Here's how the part is built. I have some questions about the finished solid (model axes, mm). Face numbers are marked on the shaded views. A direction names the side the tool comes from. Coordinates: 2 decimals unless noted, no trailing zeros. Loops run counter-clockwise (first coordinate to the right, second up) from the corner with the lowest first, then second, coordinate; pieces in that order, holes last. Notation, with made-up numbers: M 64.25,-1 L 109.25,-1 A20 cw 109.25,4 Z; hole C -39,54 d9. An arc over 180 degrees is marked long. Use CSV: the item, a comma, the result in double quotes. Start each with the question number.
Q1. If we section it at A-A (x = -6.35): Please give me the cut outline in (y, z) (3 decimals), and give its area (3 significant figures).
Q2. If we section it at C-C (x = -2): Please give me the cut outline in (y, z) (3 decimals).
Q3. If we mould it in two halves opening along Z, with no side actions, what happens to the marked faces 1, 2 and 3? For each: +Z half, -Z half, draft (parallel to the pull), parting line (faces both ways), or undercut.
Q4. If we section it at D-D (x = 8.5): Please give me the cut outline in (y, z) (3 decimals).
Q5. For pin 1 Ø5 at (x, y) = (12.7, 11.11) entering from -Z (3 decimals); pin 2 Ø3 at (x, z) = (10.5, 1.5) entering from -Y; pin 3 Ø4 at (x, z) = (-8, 2) entering from -Y, each with a flat end and sliding along its axis, tell me the tip position at first contact or that it passes through.
Q6. Which directions (+Z, -Z, +X, -X, +Y, -Y) give clear straight access to the entire face, cutting with the end or side of a thin tool? Please do the marked faces 4, 5 and 6.
Q7. Please list where these lines run through material, in increasing order: probe 1 along Z at (x, y) = (16.5, -4.5) (3 decimals); probe 2 along Y at (x, z) = (-9, 5.75); probe 3 along Y at (x, z) = (-10.5, -0.5) (3 decimals). Write a range as [from, to].
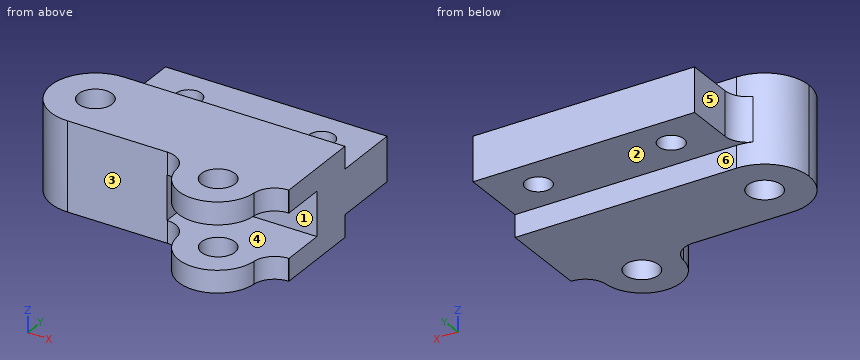
from build123d import *

# Parameters (mm, degrees)
SKETCH1_W                             = 38.1
SKETCH1_H                             = 12.699999999999998
BOSS_EXTRUDE1_DEPTH                   = 6.35
BOSS_EXTRUDE2_DEPTH                   = 3.175
F_6_CLEARANCE_HOLE1_D                 = 3.6576
F_3_16_0_1875_CLEARANCE_DOWEL_HOLE1_D = 4.826
CUT_EXTRUDE3_DEPTH                    = 3.1496
CUT_EXTRUDE3_DEPTH_BACK               = 3.175
SKETCH8_W                             = 17.4625
SKETCH8_H                             = 14.287499999999998
FILLET2_RADIUS                        = 5.55625
FILLET2_LENGTH                        = 3.2004
FILLET3_RADIUS                        = 5.55625
FILLET3_LENGTH                        = 3.175
FILLET5_R                             = 3.175
FILLET7_R                             = 6.35
FILLET8_R                             = 3.175


# Some blends are built 0.0001 mm under size
with BuildPart() as part:
    # Sketch1 → Boss-Extrude1 (new, symmetric)
    with BuildSketch(Plane.XY):
        Polygon((15.875, -14.287499999999998), (15.875, -6.349999999999994), (4.762500000000001, -6.35), (4.762500000000001, -14.287499999999996), align=None)
        Rectangle(SKETCH1_W, SKETCH1_H)
    extrude(amount=BOSS_EXTRUDE1_DEPTH, both=True)

    # Sketch2 → Boss-Extrude2 (add, symmetric)
    with BuildSketch(Plane.XY):
        Polygon((19.05, 6.35), (-12.7, 6.349999999999996), (-12.7, 15.874999999999996), (19.05, 15.875), align=None)
    extrude(amount=BOSS_EXTRUDE2_DEPTH, both=True)

    # #6 Clearance Hole1 (through all)
    with Locations(Plane.XY.offset(3.175)):
        with Locations((-6.35, 11.1125), (12.7, 11.1125)):
            Hole(F_6_CLEARANCE_HOLE1_D / 2)

    # 3/16 (0.1875) Clearance Dowel Hole1 (through all)
    with Locations(Plane.XY.offset(6.35)):
        with Locations((-12.7, 0), (10.31875, -8.5725)):
            Hole(F_3_16_0_1875_CLEARANCE_DOWEL_HOLE1_D / 2)

    # Sketch8 → Cut-Extrude3 (cut, two sides: drawn at the far end of the back side and taken through both)
    with BuildSketch(Plane.XY.offset(-CUT_EXTRUDE3_DEPTH_BACK)):
        with Locations((10.318750000000001, -7.143749999999999)):
            Rectangle(SKETCH8_W, SKETCH8_H)
    extrude(amount=CUT_EXTRUDE3_DEPTH + CUT_EXTRUDE3_DEPTH_BACK, mode=Mode.SUBTRACT)

    # Fillet2: full round fillet: the end face becomes a half cylinder, R = half its width
    fillet2_face = Plane((10.31875, -14.2875, 4.7498), x_dir=(0, 0, 1), z_dir=(0, -1, 0))  # on the end face: x along it, z out of the body
    fillet2_slab = fillet2_face.offset(-FILLET2_RADIUS / 2) * Box(FILLET2_LENGTH, 2 * FILLET2_RADIUS, FILLET2_RADIUS, mode=Mode.PRIVATE)  # the body's end, R deep
    fillet2_round = Plane((10.31875, -8.73125, 4.7498), x_dir=(0, -1, 0), z_dir=(0, 0, 1)) * Cylinder(FILLET2_RADIUS, FILLET2_LENGTH, mode=Mode.PRIVATE)  # its axis R under the face
    add(fillet2_slab - fillet2_round, mode=Mode.SUBTRACT)

    # Fillet3: full round fillet: the end face becomes a half cylinder, R = half its width
    fillet3_face = Plane((10.31875, -14.2875, -4.7625), x_dir=(0, 0, 1), z_dir=(0, -1, 0))  # on the end face: x along it, z out of the body
    fillet3_slab = fillet3_face.offset(-FILLET3_RADIUS / 2) * Box(FILLET3_LENGTH, 2 * FILLET3_RADIUS, FILLET3_RADIUS, mode=Mode.PRIVATE)  # the body's end, R deep
    fillet3_round = Plane((10.31875, -8.73125, -4.7625), x_dir=(0, -1, 0), z_dir=(0, 0, 1)) * Cylinder(FILLET3_RADIUS, FILLET3_LENGTH, mode=Mode.PRIVATE)  # its axis R under the face
    add(fillet3_slab - fillet3_round, mode=Mode.SUBTRACT)

    # Fillet5
    fillet5_edges = [part.edges().sort_by_distance(p)[0] for p in [
        (15.875, -6.349999999999997, 4.7498),
        (15.875, -6.349999999999997, -4.762499999999999),
        (4.762500000000001, -6.349999999999998, -4.762499999999999),
        (4.762500000000001, -6.349999999999998, 4.7498),
    ]]
    fillet(fillet5_edges, radius=FILLET5_R - 0.0001)  # a hair under: the kernel refuses the full size

    # Fillet7
    fillet7_edges = [part.edges().sort_by_distance(p)[0] for p in [
        (-19.05, -6.35, 0),
        (-19.05, 6.35, 0),
    ]]
    fillet(fillet7_edges, radius=FILLET7_R - 0.0001)  # a hair under: the kernel refuses the full size

    # Fillet8
    # the kernel refuses this fillet: 3.175 mm, written as the material it adds along each edge
    with BuildSketch(Plane(origin=(-12.7, 6.349999999999996, 3.175), x_dir=(-0.9856005187452213, -0.16909055990548677, 0), z_dir=(0, 0, -1))) as fillet8_piece_1:
        with BuildLine():
            CenterArc((2.6845252143088953, 3.1292731923549355), FILLET8_R, 189.73494650787575, 70.5292047157078)
            Line((-0.4447564327071806, 2.5924106646550134), (-0.7576845974087891, 2.5387244118850214))
            Line((-0.7576845974087891, 2.5387244118850214), (-0.3129281647016085, -0.05368625276999218))
            Line((-0.3129281647016085, -0.05368625276999218), (0.05368625276999203, -0.31292816470160767))
            ThreePointArc((0.05368625276999203, -0.31292816470160767), (0.05378481282186907, -0.3129112556456122), (2.0939222275177753, -0.31292731923549344))
            Line((2.0939222275177753, -0.31292731923549344), (2.1476134081351503, -2e-17))
        make_face()
    extrude(amount=6.35)


solid = part.part
Results below:
1,outline,"M -6.35,-6.35 L 6.35,-6.35 L 6.35,-3.175 L 9.284,-3.175 L 9.284,3.175 L 6.35,3.175 L 6.35,6.35 L -6.35,6.35 Z; M 12.941,-3.175 L 15.875,-3.175 L 15.875,3.175 L 12.941,3.175 Z"
1,area,"199 mm^2"
2,outline,"M -6.35,-6.35 L 6.35,-6.35 L 6.35,-3.175 L 15.875,-3.175 L 15.875,3.175 L 6.35,3.175 L 6.35,6.35 L -6.35,6.35 Z"
3,face 1,"undercut"
3,face 2,"-Z half"
3,face 3,"draft"
4,outline,"M -13.981,-6.35 L -10.158,-6.35 L -10.158,-3.175 L -13.981,-3.175 Z; M -13.981,3.15 L -10.158,3.15 L -10.158,6.35 L -13.981,6.35 Z; M -6.987,-6.35 L 6.35,-6.35 L 6.35,-3.175 L 15.875,-3.175 L 15.875,3.175 L 6.35,3.175 L 6.35,6.35 L -6.987,6.35 L -6.987,3.15 L 0,3.15 L 0,-3.175 L -6.987,-3.175 Z"
5,pin 1,"z = -3.175"
5,pin 2,"y = 0"
5,pin 3,"y = -6.35"
6,face 4,"+X, -Y"
6,face 5,"+Z, -Z, -X, +Y"
6,face 6,"-Z, +X, -X, +Y"
7,probe 1,"[-6.35, -3.175], [3.15, 6.35]"
7,probe 2,"[-6.35, 6.35]"
7,probe 3,"[-6.35, -0.991], [0.991, 15.875]"
